Input: dimensioned drawing with shaded views. Units: mm. Origin: part minimum x, y, z. A direction names the side the tool comes from. Round coordinates to 2 decimals unless told otherwise and drop trailing zeros. Write each loop counter-clockwise with the first axis right and the second up, starting at its lowest first coordinate (ties: lowest second). Pieces come first, ordered by that corner, then holes. Notation, with made-up numbers: M -7.75,58.25 L 35.25,58.25 A19 cw 35.25,93.25 Z; hole C -24.75,4.5 d6. An arc over 180 degrees is marked long. Use one line per item in the form item = value. Start each with the question number.
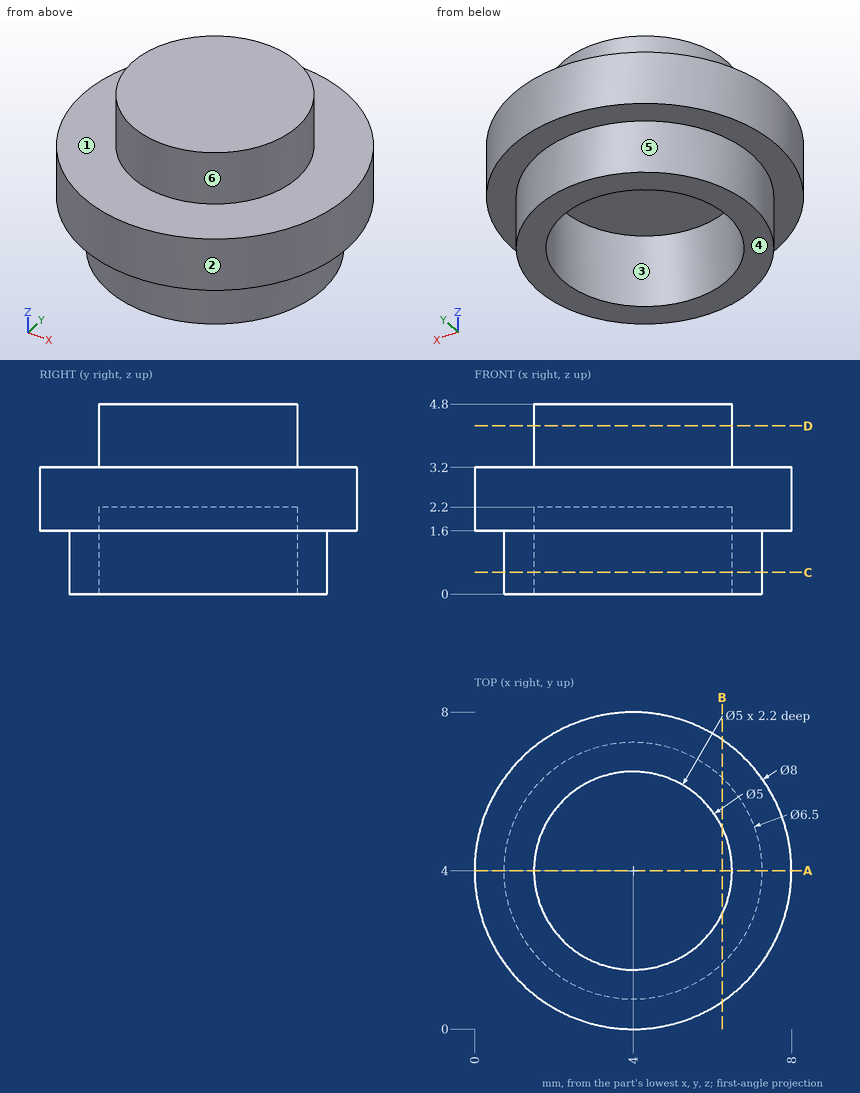
1. Section query B-B (x = 6.25). Return loops of the section in (y, z).
2. Ray query, probe 1 along Y at (x, z) = (4, 0.5); probe 2 along Y at (x, z) = (4, 1.75); probe 3 along Z at (x, y) = (6.5, 2). Return the intervals inside material, ascending.
3. Section query C-C (z = 0.55). Return loops of the section in (x, y), then the cut area to 3 significant figures.
4. Contact query for flat-ended pins moving along their axis: pin 1 (1 mm diameter, centred on y = 6.5, z = 1.5, fed in from -X); pin 2 (2 mm diameter, centred on y = 2.5, z = 4, fed in from +X); pin 3 (1.5 mm diameter, centred on y = 3, z = 4, fed in from +X). Output: stop coordinate, or through.
5. Section query A-A (y = 4). Return loops of the section in (x, z), then the cut area to 3 significant figures.
6. Section query D-D (z = 4.25). Return loops of the section in (x, y).
7. Pull-direction query (X, two-part tool) for the marked faces 1, 2 and 3; classes: released by +X, released by -X, zero draft, split by the parting line, or undercut.
8. Set-up query: the marked faces 4, 5 and 6. Return all of +Z, -Z, +X, -X, +Y, -Y with unobstructed straight access to the full face (end or side cutting, diameter ignored); none if empty.
Checks:
q1.outline = M 0.69,1.6 L 1.65,1.6 L 1.65,0 L 2.91,0 L 2.91,2.2 L 5.09,2.2 L 5.09,0 L 6.35,0 L 6.35,1.6 L 7.31,1.6 L 7.31,3.2 L 5.09,3.2 L 5.09,4.8 L 2.91,4.8 L 2.91,3.2 L 0.69,3.2 Z
q2.probe_1 = 0.75 to 1.5, 6.5 to 7.25
q2.probe_2 = 0 to 1.5, 6.5 to 8
q2.probe_3 = 0 to 3.2
q3.outline = C 4,4 d6.5; hole C 4,4 d5
q3.area = 13.5 mm^2
q4.pin_1 = 0.54
q4.pin_2 = 7.9
q4.pin_3 = 6.49
q5.outline = M 0,1.6 L 0.75,1.6 L 0.75,0 L 1.5,0 L 1.5,2.2 L 6.5,2.2 L 6.5,0 L 7.25,0 L 7.25,1.6 L 8,1.6 L 8,3.2 L 6.5,3.2 L 6.5,4.8 L 1.5,4.8 L 1.5,3.2 L 0,3.2 Z
q5.area = 20.2 mm^2
q6.outline = C 4,4 d5
q7.face_1 = zero draft
q7.face_2 = split by the parting line
q7.face_3 = undercut
q8.face_4 = -Z, +X, -X, +Y, -Y
q8.face_5 = -Z
q8.face_6 = +Z
